Could you check a few things on this model? Use its own coordinates, in mm. A direction names the side the tool comes from. Give positions to 0.01 mm unless a question says otherwise; leave off trailing zeros. Loops run counter-clockwise (first coordinate to the right, second up) from the corner with the lowest first, then second, coordinate; pieces in that order, holes last. Notation, with made-up numbers: M 1,-35 L 45,-35 A33 cw 45,-1 Z; hole C -20,30 d6. An arc over 180 degrees is marked long. Answer in a Markdown table with one row per item. Add a question column.
```python
from build123d import *

# Parameters (mm, degrees)
SKETCH_1_W          = 385
SKETCH_1_H          = 385
SKETCH_1_W_2        = 285
SKETCH_1_H_2        = 285
EXTRUDE_1_DEPTH     = 2
FILLET_1_R          = 70
FILLET_2_R          = 20
CUT_EXTRUDE_1_REACH = 546.476
SKETCH_2_R          = 1.5


with BuildPart() as part:
    # 草图1 → 凸台-拉伸1 (new body)
    with BuildSketch(Plane(origin=(0, 0, 0), x_dir=(1, 0, 0), z_dir=(0, 1, 0))):
        with Locations((192.5, 192.5)):
            Rectangle(SKETCH_1_W, SKETCH_1_H)
        with Locations((192.5, 192.5)):
            Rectangle(SKETCH_1_W_2, SKETCH_1_H_2, mode=Mode.SUBTRACT)
    extrude(amount=EXTRUDE_1_DEPTH)

    # 圆角1
    fillet_1_edges = [part.edges().sort_by_distance(p)[0] for p in [
        (0, 1, -385),
        (385, 1, -385),
        (385, 1, 0),
        (0, 1, 0),
    ]]
    fillet(fillet_1_edges, radius=FILLET_1_R)

    # 圆角2
    fillet_2_edges = [part.edges().sort_by_distance(p)[0] for p in [
        (50, 1, -335),
        (50, 1, -50),
        (335, 1, -50),
        (335, 1, -335),
    ]]
    fillet(fillet_2_edges, radius=FILLET_2_R)

    # 草图2 → 切除-拉伸1 (cut, up to next)
    with BuildSketch(Plane(origin=(0, 2, 0), x_dir=(1, 0, 0), z_dir=(0, 1, 0)), mode=Mode.PRIVATE) as cut_extrude_1_sk1:
        with Locations(Location((45.18055198, 45.18055198, 0), (0, 0, 270))):
            Circle(SKETCH_2_R)
    cut_extrude_1_tool1 = extrude(cut_extrude_1_sk1.sketch, amount=-CUT_EXTRUDE_1_REACH, mode=Mode.PRIVATE) & part.part
    # 草图2 → 切除-拉伸1 (cut, up to next)
    with BuildSketch(Plane(origin=(0, 2, 0), x_dir=(1, 0, 0), z_dir=(0, 1, 0)), mode=Mode.PRIVATE) as cut_extrude_1_sk2:
        with BuildLine():
            ThreePointArc((46.68055198, 339.81944802), (45.754577129, 341.205267318), (44.119891809, 340.880108191))
            Line((44.119891809, 340.880108191), (46.241212152, 338.758787848))
            ThreePointArc((46.241212152, 338.758787848), (46.566371279, 339.245422871), (46.68055198, 339.81944802))
        make_face()
    cut_extrude_1_tool2 = extrude(cut_extrude_1_sk2.sketch, amount=-CUT_EXTRUDE_1_REACH, mode=Mode.PRIVATE) & part.part
    # 草图2 → 切除-拉伸1 (cut, up to next)
    with BuildSketch(Plane(origin=(0, 2, 0), x_dir=(1, 0, 0), z_dir=(0, 1, 0)), mode=Mode.PRIVATE) as cut_extrude_1_sk3:
        with BuildLine():
            Line((46.241212152, 338.758787848), (44.119891809, 340.880108191))
            ThreePointArc((44.119891809, 340.880108191), (44.119891809, 338.758787848), (46.241212152, 338.758787848))
        make_face()
    cut_extrude_1_tool3 = extrude(cut_extrude_1_sk3.sketch, amount=-CUT_EXTRUDE_1_REACH, mode=Mode.PRIVATE) & part.part
    # 草图2 → 切除-拉伸1 (cut, up to next)
    with BuildSketch(Plane(origin=(0, 2, 0), x_dir=(1, 0, 0), z_dir=(0, 1, 0)), mode=Mode.PRIVATE) as cut_extrude_1_sk4:
        with BuildLine():
            ThreePointArc((46.68055198, 339.81944802), (45.754577129, 341.205267318), (44.119891809, 340.880108191))
            Line((44.119891809, 340.880108191), (46.241212152, 338.758787848))
            ThreePointArc((46.241212152, 338.758787848), (46.566371279, 339.245422871), (46.68055198, 339.81944802))
        make_face()
    cut_extrude_1_tool4 = extrude(cut_extrude_1_sk4.sketch, amount=-CUT_EXTRUDE_1_REACH, mode=Mode.PRIVATE) & part.part
    # 草图2 → 切除-拉伸1 (cut, up to next)
    with BuildSketch(Plane(origin=(0, 2, 0), x_dir=(1, 0, 0), z_dir=(0, 1, 0)), mode=Mode.PRIVATE) as cut_extrude_1_sk5:
        with BuildLine():
            Line((46.241212152, 338.758787848), (44.119891809, 340.880108191))
            ThreePointArc((44.119891809, 340.880108191), (44.119891809, 338.758787848), (46.241212152, 338.758787848))
        make_face()
    cut_extrude_1_tool5 = extrude(cut_extrude_1_sk5.sketch, amount=-CUT_EXTRUDE_1_REACH, mode=Mode.PRIVATE) & part.part
    # 草图2 → 切除-拉伸1 (cut, up to next)
    with BuildSketch(Plane(origin=(0, 2, 0), x_dir=(1, 0, 0), z_dir=(0, 1, 0)), mode=Mode.PRIVATE) as cut_extrude_1_sk6:
        with Locations(Location((339.81944802, 339.81944802, 0), (0, 0, 270))):
            Circle(SKETCH_2_R)
    cut_extrude_1_tool6 = extrude(cut_extrude_1_sk6.sketch, amount=-CUT_EXTRUDE_1_REACH, mode=Mode.PRIVATE) & part.part
    # 草图2 → 切除-拉伸1 (cut, up to next)
    with BuildSketch(Plane(origin=(0, 2, 0), x_dir=(1, 0, 0), z_dir=(0, 1, 0)), mode=Mode.PRIVATE) as cut_extrude_1_sk7:
        with Locations(Location((339.81944802, 45.18055198, 0), (0, 0, 270))):
            Circle(SKETCH_2_R)
    cut_extrude_1_tool7 = extrude(cut_extrude_1_sk7.sketch, amount=-CUT_EXTRUDE_1_REACH, mode=Mode.PRIVATE) & part.part
    add(cut_extrude_1_tool1.solids().sort_by_distance((45.180552, 2, -45.180552))[0], mode=Mode.SUBTRACT)
    add(cut_extrude_1_tool2.solids().sort_by_distance((45.63071, 2, -340.269606))[0], mode=Mode.SUBTRACT)
    add(cut_extrude_1_tool3.solids().sort_by_distance((44.730394, 2, -339.36929))[0], mode=Mode.SUBTRACT)
    add(cut_extrude_1_tool4.solids().sort_by_distance((45.63071, 2, -340.269606))[0], mode=Mode.SUBTRACT)
    add(cut_extrude_1_tool5.solids().sort_by_distance((44.730394, 2, -339.36929))[0], mode=Mode.SUBTRACT)
    add(cut_extrude_1_tool6.solids().sort_by_distance((339.819448, 2, -339.819448))[0], mode=Mode.SUBTRACT)
    add(cut_extrude_1_tool7.solids().sort_by_distance((339.819448, 2, -45.180552))[0], mode=Mode.SUBTRACT)


solid = part.part
```
Item 1: For P1, Ø4, axis at x = 339.82, z = -45.18, coming from the +Y side; P2, Ø2.5, axis at x = 45.18, z = -45.18, coming from the +Y side, each with a flat end and sliding along its axis, tell me the tip position at first contact or that it passes through.
Item 2: For faces 4 (the face through (328.986, 1.014, -55.703)), 5 (the face through (19.96, 1.01, -363.95)), which set-ups out of +Z, -Z, +X, -X, +Y, -Y let a thin tool reach every point of the face, with its end or its side?
Item 3: Suppose I cut it at A-A (z = -202.5). List the corners of the cut face in (x, y) for me.
Item 4: If we mould it in two halves opening along X, with no side actions, what happens to faces 1 (the face through (363.95, 1.01, -19.96)), 2 (the face through (19.96, 1.01, -21.05)), 3 (the face through (56.014, 1.014, -55.703))? For each: +X half, -X half, draft (parallel to the pull), parting line (faces both ways), or undercut.
Item 5: Suppose I cut it at D-D (x = 30). List the corners of the cut face in (y, z) for me.
Item 6: I need wall thicknesses on L1, parallel to Z at x = 220, y = 0.95; L2, parallel to X at y = 0.9, z = -69; L3, parallel to X at y = 0.2, z = -44. Which ranges of each line are inside material? Lowest first, please.
Item 7: Suppose I cut it at B-B (x = 299.5). List the corners of the cut face in (y, z) for me, then the cut area to 3 significant figures.
Item 8: Suppose I cut it at C-C (y = 1.35). List the corners of the cut face in (x, z) for me, then the cut area to 3 significant figures.
Values found:
| question | item | result |
|---|---|---|
| 1 | P1 | y = 2 |
| 1 | P2 | through |
| 2 | face 4 | +Y, -Y |
| 2 | face 5 | -Z, -X, +Y, -Y |
| 3 | outline | M 0,0 L 50,0 L 50,2 L 0,2 Z; M 335,0 L 385,0 L 385,2 L 335,2 Z |
| 4 | face 1 | +X half |
| 4 | face 2 | -X half |
| 4 | face 3 | undercut |
| 5 | outline | M 0,-372.45 L 2,-372.45 L 2,-12.55 L 0,-12.55 Z |
| 6 | L1 | -385 to -335, -50 to 0 |
| 6 | L2 | 0.01 to 50.03, 334.97 to 384.99 |
| 6 | L3 | 5.01 to 44.26, 46.11 to 338.89, 340.74 to 379.99 |
| 7 | outline | M 0,-385 L 2,-385 L 2,-335 L 0,-335 Z; M 0,-50 L 2,-50 L 2,0 L 0,0 Z |
| 7 | area | 200 mm² |
| 8 | outline | M 0,-315 A70 ccw 70,-385 L 315,-385 A70 ccw 385,-315 L 385,-70 A70 ccw 315,0 L 70,0 A70 ccw 0,-70 Z; hole C 45.18,-339.82 d3; hole C 45.18,-45.18 d3; hole M 50,-315 A20 ccw 70,-335 L 315,-335 A20 ccw 335,-315 L 335,-70 A20 ccw 315,-50 L 70,-50 A20 ccw 50,-70 Z; hole C 339.82,-339.82 d3; hole C 339.82,-45.18 d3 |
| 8 | area | 63,100 mm² |
